Geometry: final body of the model. Coordinates: model frame, mm. A direction names the side the tool comes from. Give positions to 0.01 mm unless a question says otherwise; leave off trailing zeros. Write each loop counter-clockwise with the first axis right and the second up, starting at its lowest first coordinate (ties: lowest second). Pieces come first, ordered by that corner, then holes. Notation, with made-up numbers: M 85.25,-38 L 119.25,-38 A29 ccw 119.25,-1 Z; hole C 75.5,3.25 d10. An arc over 180 degrees is marked long. Use a Markdown table: item, result. Add a question column.
(1) Cut plane D-D (x = 55). Output: boundary loops of the cut face in (y, z), plus the area to 3 significant figures.
(2) Reachability of faces 1 (the flat face through (41.529, -3, -28)), 2 (the cylindrical face through (64.756, -3.131, -70.768)), 3 (the flat face through (-47, -3, -57.15)), 4 (the flat face through (32, -3, 50.8)) from +Z, -Z, +X, -X, +Y, -Y: full face, straight path, thin tool, end or side. Return the list, or none.
(3) Cut plane A-A (y = -2.25). Output: boundary loops of the cut face in (x, z) (3 decimals), plus the area to 3 significant figures.
(4) Draft query along X for faces 5 (the flat face through (-41.529, -3, -20)), 6 (the flat face through (-1, -3, 19.05)), 7 (the flat face through (-1, 0, 35)), 8 (the cylindrical face through (7.625, -3.131, 52.611)). Return one class per face: released by +X, released by -X, zero draft, split by the parting line, or undercut.
(5) Material intervals for L1, parallel to X at y = -2, z = -25.5 (3 decimals); L2, parallel to Z at x = 38, y = -2.5; L3, parallel to Z at x = -45, y = -5.5, sorted ascending.
(6) Cut plane C-C (x = 14.5). Output: boundary loops of the cut face in (y, z), plus the area to 3 significant figures.
(7) Pin query (flat end, axial travel): pin 1 Ø1.9 at (x, y) = (11.5, -1.5) entering from -Z; pin 2 Ø3 at (x, y) = (28.5, -3.5) entering from +Z. Return the tip coordinate at first contact, or that it passes through.
(8) Cut plane B-B (z = 4.5). Output: boundary loops of the cut face in (x, y) (3 decimals), plus the area to 3 significant figures.
```python
from build123d import *

# Parameters (mm, degrees)
F0_R     = 6.477
F1_DEPTH = 6.35


with BuildPart() as f1:
    # F0 (on Front) → F1 (new body)
    with BuildSketch(Plane.XZ):
        with BuildLine():
            Line((41.529, -76.2), (51.435, -76.2))
            ThreePointArc((51.435, -76.2), (64.905384, -70.620384), (70.485, -57.15))
            Line((70.485, -57.15), (70.485, 31.75))
            ThreePointArc((70.485, 31.75), (64.905384, 45.220384), (51.435, 50.8))
            Line((51.435, 50.8), (12.065, 50.8))
            ThreePointArc((12.065, 50.8), (7.574872, 52.659872), (5.715, 57.15))
            ThreePointArc((5.715, 57.15), (0.135384, 70.620384), (-13.335, 76.2))
            Line((-13.335, 76.2), (-51.435, 76.2))
            ThreePointArc((-51.435, 76.2), (-64.905384, 70.620384), (-70.485, 57.15))
            Line((-70.485, 57.15), (-70.485, -38.1))
            ThreePointArc((-70.485, -38.1), (-64.905384, -51.570384), (-51.435, -57.15))
            Line((-51.435, -57.15), (-41.529, -57.15))
            Line((-41.529, -57.15), (-41.529, 19.05))
            Line((-41.529, 19.05), (41.529, 19.05))
            Line((41.529, 19.05), (41.529, -76.2))
        make_face()
        with Locations((-32.385, 57.15)):
            Circle(F0_R, mode=Mode.SUBTRACT)
    extrude(amount=F1_DEPTH)


solid = f1.part
```
Answer list:
| question | item | result |
|---|---|---|
| 1 | outline | M -6.35,-75.86 L 0,-75.86 L 0,50.46 L -6.35,50.46 Z |
| 1 | area | 802 mm² |
| 2 | face 1 | -Z, +Y, -Y |
| 2 | face 2 | -Z, +X, +Y, -Y |
| 2 | face 3 | -Z, -X, +Y, -Y |
| 2 | face 4 | +Z, +X, +Y, -Y |
| 3 | outline | M -70.485,-38.1 A19.05 ccw -51.435,-57.15 L -41.529,-57.15 L -41.529,19.05 L 41.529,19.05 L 41.529,-76.2 L 51.435,-76.2 A19.05 ccw 70.485,-57.15 L 70.485,31.75 A19.05 ccw 51.435,50.8 L 12.065,50.8 A6.35 cw 5.715,57.15 A19.05 ccw -13.335,76.2 L -51.435,76.2 A19.05 ccw -70.485,57.15 Z; hole C -32.385,57.15 d12.954 |
| 3 | area | 10,900 mm² |
| 4 | face 5 | undercut |
| 4 | face 6 | undercut |
| 4 | face 7 | zero draft |
| 4 | face 8 | released by +X |
| 5 | L1 | -70.485 to -41.529, 41.529 to 70.485 |
| 5 | L2 | 19.05 to 50.8 |
| 5 | L3 | -57.15 to 76.2 |
| 6 | outline | M -6.35,19.05 L 0,19.05 L 0,50.8 L -6.35,50.8 Z |
| 6 | area | 202 mm² |
| 7 | pin 1 | z = 19.05 |
| 7 | pin 2 | z = 50.8 |
| 8 | outline | M -70.485,-6.35 L -41.529,-6.35 L -41.529,0 L -70.485,0 Z; M 41.529,-6.35 L 70.485,-6.35 L 70.485,0 L 41.529,0 Z |
| 8 | area | 368 mm² |
